Geometry check sheet. Reference: the model listing, model coordinates, mm. A direction names the side the tool comes from. Round coordinates to 2 decimals unless told otherwise and drop trailing zeros. Order: outer loops, then holes, each group sorted by start corner. A loop starts at its lowest first (then second) coordinate and runs counter-clockwise, first axis right, second up.
(1) Go/stop test with flat-tipped pins: pin 1 (3 mm diameter, centred on y = 10.5, z = -30.5, fed in from -X); pin 2 (4 mm diameter, centred on y = 3.5, z = -116, fed in from +X). Record where each tip stops, or that it passes through.
(2) Material ranges on line 1 along X through (y, z) = (10.75, -37); line 2 along X through (y, z) = (1.25, -93); line 3 along Z through (x, y) = (-45.5, 10.5), recorded low to high.
(3) Sectioned sample at B-B (z = -29.5). Record the boundary of the cut face in (x, y), plus the area to 3 significant figures.
(4) Sectioned sample at C-C (x = -94.5). Record the boundary of the cut face in (y, z), plus the area to 3 significant figures.
(5) Set-up check for faces 5 (the face through (-146.5, 6, -140)), 6 (the face through (-150, 6, -157)): record each of +Z, -Z, +X, -X, +Y, -Y from which the full face is reachable in a straight line by a thin tool's end or side.
(6) Sectioned sample at A-A (y = 9.5). Record the boundary of the cut face in (x, z), plus the area to 3 significant figures.
(7) Release check for a two-part mould opening along Z. For faces 1 (the face through (-148, 6, -152)), 2 (the face through (-146.5, 6, -29)), 3 (the face through (-150, 6, -84)), 4 (the face through (-73, 6, -88)) record: +Z half, -Z half, draft (parallel to the pull), parting line (faces both ways), or undercut.
Autodesk Inventor part; units mm, degrees
ref_plane "YZ Plane" through (0, 0, 0) normal (1, 0, 0) x (0, 1, 0)
ref_plane "XZ Plane" through (0, 0, 0) normal (0, 1, 0) x (-1, 0, 0)
ref_plane "XY Plane" through (0, 0, 0) normal (0, 0, 1) x (1, 0, 0)
sketch "Sketch1" plane through (0, 0, 0) normal (0, 1, 0) x (-1, 0, 0)
  line L0 (0, -12) -> (150, -12)
  line L1 (150, -12) -> (-170, -12)
  line L2 (150, -12) -> (150, 0)
  line L3 (-170, 0) -> (150, 0)
  line L4 (-170, -12) -> (-170, 0)
  arc A0 (0, -37) -> (21.03, -61.6828) centre (25, -37) ccw
  line L5 (0, -12) -> (0, -37)
  arc A1 (100.3172, -140.97) -> (125, -162) centre (125, -137) ccw
  line L6 (150, -162) -> (125, -162)
  arc A2 (100.3172, -140.97) -> (21.03, -61.6828) centre (5.8332, -156.1668) ccw
  line L7 (150, -17) -> (146.5, -17)
  line L8 (146.5, -17) -> (146.5, -41.5)
  line L9 (146.5, -41.5) -> (150, -41.5)
  line L10 (150, -127.5) -> (146.5, -127.5)
  line L11 (146.5, -127.5) -> (146.5, -152)
  line L12 (146.5, -152) -> (150, -152)
  line L13 (150, -12) -> (150, -17)
  line L14 (150, -41.5) -> (150, -127.5)
  line L15 (150, -152) -> (150, -162)
  line L16 (162.5, -20.3274) -> (147.5, -20.3274)
  line L17 (147.5, -37.698) -> (162.5, -37.698)
  line L18 (147.5, -40.746) -> (162.5, -40.746)
  line L19 (162.246, -41) -> (147.754, -41)
  line L20 (147.754, -17) -> (162.246, -17)
  line L21 (162.5, -17.254) -> (147.5, -17.254)
  line L22 (147.5, -20.3274) -> (147.5, -37.698) construction
  point P0 (0, 0)
extrude "Tykkelse af plade" add sketch "Sketch1" along normal blind 12 contours L0 L13 L7 L8 L9 L14 L10 L11 L12 L15 L6 A1 A2 A0 L5
equation "\"d12\" = d9"
equation "\"d13\" = d16"
properties part number "Z Holdere" material "Wood (Cherry)"
Answer below:
1. pin 1: stops at x = -146.5
1. pin 2: stops at x = -91.74
2. line 1: x = -146.5 to 0
2. line 2: x = -150 to -77.72
2. line 3: z = -69.08 to -12
3. outline: (-146.5, 0) - (0, 0) - (0, 12) - (-146.5, 12) - close
3. area: 1,760 mm2
4. outline: (0, -120.16) - (12, -120.16) - (12, -12) - (0, -12) - close
4. area: 1,300 mm2
5. face 5: -X, +Y, -Y
5. face 6: +Z, -Z, -X, +Y, -Y
6. outline: (-150, -162) - (-125, -162) arc R25 ccw to (-100.32, -140.97) arc R95.7 cw to (-21.03, -61.68) arc R25 ccw to (0, -37) - (0, -12) - (-150, -12) - (-150, -17) - (-146.5, -17) - (-146.5, -41.5) - (-150, -41.5) - (-150, -127.5) - (-146.5, -127.5) - (-146.5, -152) - (-150, -152) - close
6. area: 13,800 mm2
7. face 1: undercut
7. face 2: undercut
7. face 3: draft
7. face 4: -Z half
